Check sheet for the modelled part. Datum: model origin and axes. Units: mm. Face numbers are marked on the shaded views. A direction names the side the tool comes from. Coordinates: 2 decimals unless noted, no trailing zeros. Write each loop counter-clockwise with the first axis right and the second up, starting at its lowest first coordinate (ties: lowest second). Pieces come first, ordered by that corner, then holes. Notation, with made-up numbers: (-26.75, 89) -> (30.25, 89) arc R32 cw to (30.25, 128) -> close; hole circle Ø1 at (66.5, 21). An arc over 180 degrees is marked (long way). One line per item, written item: value. Start each with the question number.
1) Sectioned sample at B-B on x = 13. Enter the section's corners in (y, z), plus the area to 3 significant figures.
2) Gauge pin test, flat ends, axial feed: P1, Ø1.6, axis at x = -14, z = 5.5, coming from the +Y side; P2, Ø1, axis at y = 5, z = 1.5, coming from the +X side. Record the tip position at first contact, or that the pin passes through.
3) Sectioned sample at D-D on z = 5. Give the number of separate pieces and of enclosed holes in the cut face, plus the area to 3 significant figures.
4) Scan lines: line 1 along X through (y, z) = (17.75, 5); line 2 along X through (y, z) = (12, 3.5) (3 decimals); line 3 along Y through (x, z) = (0, 4.25). Record each from-to range of solid material in increasing order. Write a range as [from, to].
5) Set-up check for the marked faces 4, 5 and 6: record each of +Z, -Z, +X, -X, +Y, -Y from which the full face is reachable in a straight line by a thin tool's end or side.
6) Sectioned sample at C-C on y = 0. Enter the section's corners in (x, z), plus the area to 3 significant figures.
7) Sectioned sample at A-A on y = -10. Enter the section's corners in (x, z) (3 decimals), plus the area to 3 significant figures.
8) Draft check along X on the marked faces 1, 2 and 3. Enter one of: +X half, -X half, draft (parallel to the pull), parting line (faces both ways), or undercut.
```python
from build123d import *

# Parameters (mm, degrees)
SKETCH1_W                                  = 35
SKETCH1_H                                  = 38.1
BOSS_EXTRUDE1_DEPTH                        = 10
F_3_3_3_3_DIAMETER_HOLE1_D                 = 3.3
SKETCH4_R                                  = 3.2
CUT_EXTRUDE1_DEPTH                         = 28.733598757
SKETCH5_W                                  = 8
SKETCH5_H                                  = 9.05
CUT_EXTRUDE2_DEPTH                         = 10
CUT_EXTRUDE3_DEPTH                         = 3
MIRROR2_AT_THE_SECOND_PLANE_COPY_1_SKETC_W = 8
MIRROR2_AT_THE_SECOND_PLANE_COPY_1_SKETC_H = 9.05
MIRROR2_AT_THE_SECOND_PLANE_COPY_1_DEPTH   = 10
MIRROR2_AT_THE_SECOND_PLANE_COPY_2_DEPTH   = 3
CUT_EXTRUDE4_DEPTH                         = 28.733598757
CUT_EXTRUDE4_DEPTH_BACK                    = 28.733598757
SKETCH7_W                                  = 1
SKETCH7_H                                  = 1


with BuildPart() as part:
    # Sketch1 → Boss-Extrude1 (new body)
    with BuildSketch(Plane.XY):
        Rectangle(SKETCH1_W, SKETCH1_H)
    extrude(amount=BOSS_EXTRUDE1_DEPTH)

    # Ø3.3 (3.3) Diameter Hole1 (through all)
    with Locations(Plane(origin=(0, 19.05, 0), x_dir=(1, 0, 0), z_dir=(0, 1, 0))):
        with Locations((-13.47, -5), (13.47, -5)):
            Hole(F_3_3_3_3_DIAMETER_HOLE1_D / 2)

    # Sketch4 → Cut-Extrude1 (cut, through all)
    with BuildSketch(Plane.XY.offset(10)):
        Circle(SKETCH4_R)
    extrude(amount=-CUT_EXTRUDE1_DEPTH, mode=Mode.SUBTRACT)

    # Sketch5 → Cut-Extrude2 (cut)
    with BuildSketch(Plane(origin=(0, 0, 0), x_dir=(-1, 0, 0), z_dir=(0, 0, -1))):
        with Locations((-13.5, 4.525)):
            Rectangle(SKETCH5_W, SKETCH5_H)
    cut_extrude2 = extrude(amount=-CUT_EXTRUDE2_DEPTH, mode=Mode.SUBTRACT)

    # Sketch6 → Cut-Extrude3 (cut)
    with BuildSketch(Plane.XZ.offset(-9.05)):
        Polygon((16.195, 6.573279484), (13.47, 8.146558967), (10.745, 6.573279484), (10.745, 3.426720516), (13.47, 1.853441033), (16.195, 3.426720516), align=None)
    cut_extrude3 = extrude(amount=-CUT_EXTRUDE3_DEPTH, mode=Mode.SUBTRACT)

    # Mirror2: Cut-Extrude2, Cut-Extrude3 across plane
    add(cut_extrude2.mirror(Plane(origin=(0, 0, 0), x_dir=(0, 0, 1), z_dir=(1, 0, 0))), mode=Mode.SUBTRACT)
    add(cut_extrude3.mirror(Plane(origin=(0, 0, 0), x_dir=(0, 0, 1), z_dir=(1, 0, 0))), mode=Mode.SUBTRACT)

    # Mirror2 at the second plane: Cut-Extrude2, Cut-Extrude3 across plane
    add(cut_extrude2.mirror(Plane.ZX), mode=Mode.SUBTRACT)
    add(cut_extrude3.mirror(Plane.ZX), mode=Mode.SUBTRACT)

    # Mirror2 at the second plane copy 1 sketc → Mirror2 at the second plane copy 1 (cut)
    with BuildSketch(Plane(origin=(0, 0, 0), x_dir=(1, 0, 0), z_dir=(0, 0, -1))):
        with Locations((-13.5, 4.525)):
            Rectangle(MIRROR2_AT_THE_SECOND_PLANE_COPY_1_SKETC_W, MIRROR2_AT_THE_SECOND_PLANE_COPY_1_SKETC_H)
    extrude(amount=-MIRROR2_AT_THE_SECOND_PLANE_COPY_1_DEPTH, mode=Mode.SUBTRACT)

    # Mirror2 at the second plane copy 2 sketc → Mirror2 at the second plane copy 2 (cut)
    with BuildSketch(Plane(origin=(0, -9.05, 0), x_dir=(-1, 0, 0), z_dir=(0, 1, 0))):
        Polygon((16.195, 6.573279484), (13.47, 8.146558967), (10.745, 6.573279484), (10.745, 3.426720516), (13.47, 1.853441033), (16.195, 3.426720516), align=None)
    extrude(amount=-MIRROR2_AT_THE_SECOND_PLANE_COPY_2_DEPTH, mode=Mode.SUBTRACT)

    # Sketch7 → Cut-Extrude4 (cut, two sides: drawn at the far end of the back side and taken through both)
    with BuildSketch(Plane.XY.offset(10).offset(-CUT_EXTRUDE4_DEPTH_BACK)):
        with Locations((0, 3.660696126)):
            Rectangle(SKETCH7_W, SKETCH7_H)
    extrude(amount=CUT_EXTRUDE4_DEPTH + CUT_EXTRUDE4_DEPTH_BACK, mode=Mode.SUBTRACT)


solid = part.part
```
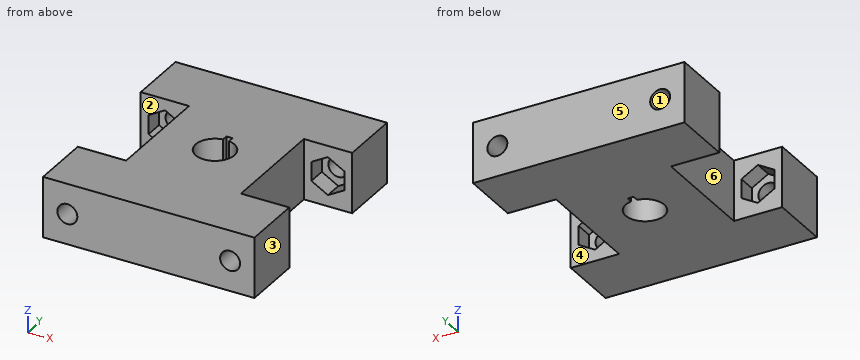
Answers:
1. outline: (-19.05, 0) -> (-9.05, 0) -> (-9.05, 2.12) -> (-12.05, 2.12) -> (-12.05, 3.42) -> (-19.05, 3.42) -> close; (-19.05, 6.58) -> (-12.05, 6.58) -> (-12.05, 7.88) -> (-9.05, 7.88) -> (-9.05, 10) -> (-19.05, 10) -> close; (9.05, 0) -> (19.05, 0) -> (19.05, 3.42) -> (12.05, 3.42) -> (12.05, 2.12) -> (9.05, 2.12) -> close; (9.05, 7.88) -> (12.05, 7.88) -> (12.05, 6.58) -> (19.05, 6.58) -> (19.05, 10) -> (9.05, 10) -> close
1. area: 121 mm2
2. P1: passes through
2. P2: stops at x = 9.5
3. separate pieces: 5
3. enclosed holes: 1
3. area: 853 mm2
4. line 1: x = [-17.5, -15.12], [-11.82, 11.82], [15.12, 17.5]
4. line 2: x = [-17.5, -16.195], [-10.745, 10.745], [16.195, 17.5]
4. line 3: y = [-19.05, -3.2], [4.16, 19.05]
5. face 4: +Z, -Z, +X
5. face 5: +Z, -Z, +X, -X, +Y
5. face 6: +Z, -Z, -X
6. outline: (-9.5, 0) -> (-3.2, 0) -> (-3.2, 10) -> (-9.5, 10) -> close; (3.2, 0) -> (9.5, 0) -> (9.5, 10) -> (3.2, 10) -> close
6. area: 126 mm2
7. outline: (-17.5, 0) -> (17.5, 0) -> (17.5, 10) -> (-17.5, 10) -> close; hole (-16.195, 3.427) -> (-13.47, 1.853) -> (-10.745, 3.427) -> (-10.745, 6.573) -> (-13.47, 8.147) -> (-16.195, 6.573) -> close; hole (10.745, 3.427) -> (13.47, 1.853) -> (16.195, 3.427) -> (16.195, 6.573) -> (13.47, 8.147) -> (10.745, 6.573) -> close
7. area: 299 mm2
8. face 1: undercut
8. face 2: draft
8. face 3: +X half
